Build history of the part. All positions in model axes, mm. Round coordinates to 2 decimals unless told otherwise and drop trailing zeros. Write each loop counter-clockwise with the first axis right and the second up, starting at its lowest first coordinate (ties: lowest second). Pieces come first, ordered by that corner, then holes. Notation, with made-up numbers: (-39, -26) -> (17, -26) arc R23 cw to (17, -12) -> close; hole circle Ø8 at (2.25, -20). An arc over 180 degrees is marked (long way). Answer in a Markdown table with one row per item.
```python
from build123d import *

# Parameters (mm, degrees)
SKETCH2_R           = 9
SKETCH2_R_2         = 1.5875
BOSS_EXTRUDE2_DEPTH = 5
CUT_EXTRUDE1_DEPTH  = 6
FILLET1_R           = 0.2


with BuildPart() as part:
    # Sketch2 → Boss-Extrude2 (new body)
    with BuildSketch(Plane.XY):
        with Locations((-0.284627084, 9.330933041)):
            Circle(SKETCH2_R)
        with Locations((-0.284627084, 9.330933041)):
            Circle(SKETCH2_R_2, mode=Mode.SUBTRACT)
    extrude(amount=BOSS_EXTRUDE2_DEPTH)

    # Sketch3 → Cut-Extrude1 (cut, through all)
    with BuildSketch(Plane.XY.offset(5)):
        with BuildLine():
            Line((-4.158820782, 1.20747176), (-4.158820782, 3.631161293))
            ThreePointArc((-4.158820782, 3.631161293), (-3.331539319, 5.251263522), (-1.534089549, 5.531085209))
            ThreePointArc((-1.534089549, 5.531085209), (0.362418992, 5.383613523), (2.112594321, 6.128850978))
            ThreePointArc((2.112594321, 6.128850978), (3.05528193, 6.511368207), (4.064188319, 6.380649971))
            Line((4.064188319, 6.380649971), (7.578508136, 4.952451053))
            ThreePointArc((7.578508136, 4.952451053), (2.451086916, 0.756793497), (-4.158820782, 1.20747176))
        make_face()
    extrude(amount=-CUT_EXTRUDE1_DEPTH, mode=Mode.SUBTRACT)

    # Fillet1
    fillet1_edges = [part.edges().sort_by_distance(p)[0] for p in [
        (-4.158820782, 1.20747176, 2.5),
    ]]
    fillet(fillet1_edges, radius=FILLET1_R)


solid = part.part
```
Q1. Saw through at A-A on y = 9. Write the cut outline in (x, z).
A:
| item | result |
|---|---|
| outline | (-9.28, 0) -> (-1.84, 0) -> (-1.84, 5) -> (-9.28, 5) -> close; (1.27, 0) -> (8.71, 0) -> (8.71, 5) -> (1.27, 5) -> close |
Q2. Saw through at D-D on y = 13.25. Write the cut outline in (x, z), plus the area to 3 significant figures.
A:
| item | result |
|---|---|
| outline | (-8.39, 0) -> (7.82, 0) -> (7.82, 5) -> (-8.39, 5) -> close |
| area | 81.0 mm² |
Q3. Wall check: line 1 (Y direction, x = -0.25, z = 3.4); line 2 (X direction, y = 5.25, z = 1.9); line 3 (Y direction, x = -6, z = 3.75). Give the ranges that are in metal, low to high. Write a range as [from, to].
A:
| item | result |
|---|---|
| line 1 | [5.33, 7.74], [10.92, 18.33] |
| line 2 | [-8.31, -3.33], [6.85, 7.74] |
| line 3 | [2.38, 16.28] |
Q4. Drop flat-ended pins along their axis: P1, Ø1, axis at y = 13.5, z = 2.5, coming from the +X side; P2, Ø2.5, axis at y = 2.5, z = 2.5, coming from the +X side; P3, Ø1.5, axis at x = 3, z = 2.5, coming from the +Y side. Give the stop position or say it passes through.
A:
| item | result |
|---|---|
| P1 | x = 7.93 |
| P2 | x = -4.16 |
| P3 | y = 17.97 |
Q5. Saw through at C-C on x = -7.5. Write the cut outline in (y, z), plus the area to 3 significant figures.
A:
| item | result |
|---|---|
| outline | (3.95, 0) -> (14.71, 0) -> (14.71, 5) -> (3.95, 5) -> close |
| area | 53.8 mm² |
Q6. Two-plate mould, pull along X, no slides. Class faces 1 (the cylindrical face through (-2.577, 18.034, 2.465)), 2 (the flat face through (-4.159, 3, 3)), 3 (the cylindrical face through (0.34, 5.38, 2.54)), 4 (the flat face through (5.797, 5.677, 2.535)): released by +X, released by -X, zero draft, split by the parting line, or undercut.
A:
| item | result |
|---|---|
| face 1 | split by the parting line |
| face 2 | released by +X |
| face 3 | undercut |
| face 4 | undercut |
